from build123d import *

# Parameters (mm, degrees)
BOSS_EXTRUDE1_DEPTH      = 15
BOSS_EXTRUDE1_DEPTH_BACK = 15
SKETCH1_R                = 9
SKETCH1_R_2              = 5


with BuildPart() as part:
    # Sketch1 → Boss-Extrude1 (new, two sides: drawn at the far end of the back side and taken through both)
    with BuildSketch(Plane.XY.offset(-BOSS_EXTRUDE1_DEPTH_BACK)):
        with BuildLine():
            Line((282.195121951, 33.780487805), (-6.624538161, 33.780487805))
            ThreePointArc((-6.624538161, 33.780487805), (-17.804878049, 38.780487805), (-28.985217936, 33.780487805))
            Line((-28.985217936, 33.780487805), (-67.804878049, 33.780487805))
            ThreePointArc((-67.804878049, 33.780487805), (-77.804878049, 23.780487805), (-67.804878049, 13.780487805))
            Line((-67.804878049, 13.780487805), (-28.985217936, 13.780487805))
            ThreePointArc((-28.985217936, 13.780487805), (-17.804878049, 8.780487805), (-6.624538161, 13.780487805))
            Line((-6.624538161, 13.780487805), (282.195121951, 13.780487805))
            Line((282.195121951, 13.780487805), (282.195121951, 33.780487805))
        make_face()
        with Locations((-17.804878049, 23.780487805)):
            Circle(SKETCH1_R, mode=Mode.SUBTRACT)
        with Locations((-67.804878049, 23.780487805)):
            Circle(SKETCH1_R_2, mode=Mode.SUBTRACT)
    extrude(amount=BOSS_EXTRUDE1_DEPTH + BOSS_EXTRUDE1_DEPTH_BACK)


solid = part.part
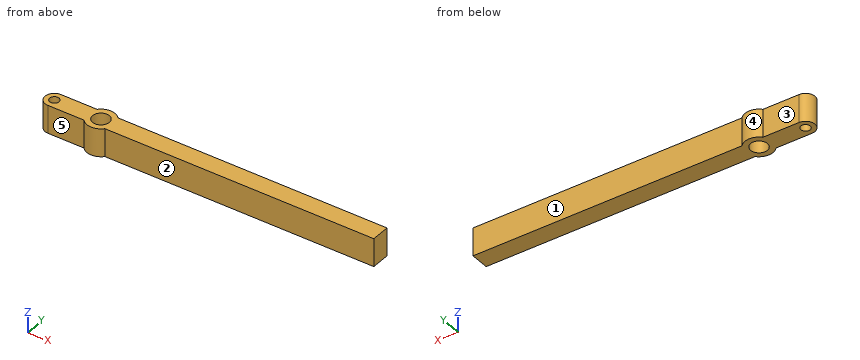
The model under review builds one solid part; all positions refer to its coordinate system, in mm. Face numbers are marked on the shaded views. A direction names the side the tool comes from. Round coordinates to 2 decimals unless told otherwise and drop trailing zeros. Write each loop counter-clockwise with the first axis right and the second up, starting at its lowest first coordinate (ties: lowest second). Pieces come first, ordered by that corner, then holes. Notation, with made-up numbers: M 50.5,47 L 66.5,47 A27 ccw 66.5,79 Z; hole C 13,-11.75 d5. An arc over 180 degrees is marked long. Use a Markdown table: item, result. Add a question column.
Q1. To check wall thickness, follow line 1 (X direction, y = 21.75, z = -7.75); line 2 (Y direction, x = 151.5, z = -12); line 3 (X direction, y = 16.5, z = 6). State the ranges of each line that lie inside material, in increasing order.
Q2. Machinability: for the marked faces 1, 2, 3, 4 and 5, which of the approach directions +Z, -Z, +X, -X, +Y, -Y give a long, thin tool a straight path to every point of the face, cutting with its end or side? Answer none if there is none.
Q3. We need section A-A, the plane z = 8.75. State the section outline as (x, y) points, plus the area to 3 significant figures.
Q4. We need section B-B, the plane x = 21.5. State the section outline as (y, z) points.
Q5. Insertion check: pin 1 (5 mm diameter, centred on x = 213.5, z = -7, fed in from +Y); pin 2 (3 mm diameter, centred on y = 20, z = 7, fed in from -X); pin 3 (5 mm diameter, centred on x = 56, z = -11, fed in from -Y); pin 4 (4 mm diameter, centred on y = 13, z = -10.5, fed in from +X). Each pin has a flat end and moves straight along its axis. Give the tip position at first contact, or say it passes through.
Findings below:
| question | item | result |
|---|---|---|
| 1 | line 1 | x = -77.6 to -72.37, -63.24 to -26.57, -9.04 to 282.2 |
| 1 | line 2 | y = 13.78 to 33.78 |
| 1 | line 3 | x = -74.66 to -23.1, -12.51 to 282.2 |
| 2 | face 1 | +Z, -Z, +X, +Y |
| 2 | face 2 | +Z, -Z, +X, -Y |
| 2 | face 3 | +Z, -Z, -X, +Y |
| 2 | face 4 | +Z, -Z, +Y |
| 2 | face 5 | +Z, -Z, -X, -Y |
| 3 | outline | M -67.8,13.78 L -28.99,13.78 A15 ccw -6.62,13.78 L 282.2,13.78 L 282.2,33.78 L -6.62,33.78 A15 ccw -28.99,33.78 L -67.8,33.78 A10 ccw Z; hole C -67.8,23.78 d10; hole C -17.8,23.78 d18 |
| 3 | area | 6,980 mm² |
| 4 | outline | M 13.78,-15 L 33.78,-15 L 33.78,15 L 13.78,15 Z |
| 5 | pin 1 | stops at y = 33.78 |
| 5 | pin 2 | stops at x = -77.54 |
| 5 | pin 3 | stops at y = 13.78 |
| 5 | pin 4 | stops at x = 282.2 |
